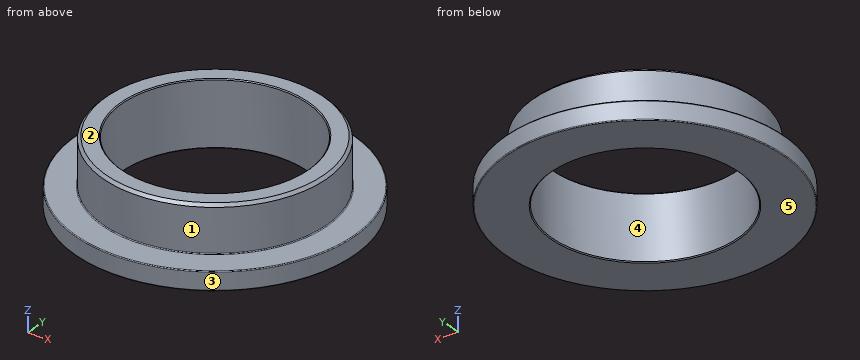
from build123d import *

# Parameters (mm, degrees)
CHAMFER1_SIZE = 0.15
CHAMFER2_SIZE = 0.05
FILLET1_R     = 0.045


with BuildPart() as part:
    # Sketch3 → Revolve1 (revolve)
    with BuildSketch(Plane(origin=(0, 0, 0), x_dir=(0, 0, -1), z_dir=(1, 0, 0))):
        Polygon((1.75, -7.5), (0.75, -7.5), (0.75, -6), (-1.75, -6), (-1.75, -5), (1.75, -5), align=None)
    revolve(axis=Axis((0, 0, 1.75), (0, 0, -1)))

    # Chamfer1
    chamfer1_edges = [part.edges().sort_by_distance(p)[0] for p in [
        (0, 6, 1.75),
    ]]
    chamfer(chamfer1_edges, length=CHAMFER1_SIZE)

    # Chamfer2
    chamfer2_edges = [part.edges().sort_by_distance(p)[0] for p in [
        (0, 5, -1.75),
        (0, 5, 1.75),
    ]]
    chamfer(chamfer2_edges, length=CHAMFER2_SIZE)

    # Fillet1
    fillet1_edges = [part.edges().sort_by_distance(p)[0] for p in [
        (0, 6, -0.75),
        (0, 7.5, -0.75),
        (0, 7.5, -1.75),
    ]]
    fillet(fillet1_edges, radius=FILLET1_R)


solid = part.part
The listing builds one solid part. Answer for the finished solid, in the listing's coordinates (mm). Face numbers are marked on the shaded views. A direction names the side the tool comes from. Give positions to 0.01 mm unless a question says otherwise; leave off trailing zeros. Order: outer loops, then holes, each group sorted by start corner. A loop starts at its lowest first (then second) coordinate and runs counter-clockwise, first axis right, second up. Notation, with made-up numbers: (-31, 45) - (-3, 45) arc R25 cw to (-3, 59) - close; hole circle Ø4 at (86.25, 65). An arc over 180 degrees is marked (long way). Use one line per item in the form item = value.
1) Find section D-D on z = -0.2. Determine the outline of the cut face in (x, y), and give its area (3 significant figures).
Verdict:
outline = circle Ø12 at (0, 0); hole circle Ø10 at (0, 0)
area = 34.6 mm^2
2) The mould has two halves that part along X. Classify the marked faces 3, 4 and 5: released by +X, released by -X, zero draft, split by the parting line, or undercut.
Verdict:
face_3 = split by the parting line
face_4 = undercut
face_5 = zero draft
3) Find section A-A on y = 0. Determine the outline of the cut face in (x, z) (3 decimals), and give its area (3 significant figures).
Verdict:
outline = (-7.5, -1.705) arc R0.045 ccw to (-7.455, -1.75) - (-5.05, -1.75) - (-5, -1.7) - (-5, 1.7) - (-5.05, 1.75) - (-5.85, 1.75) - (-6, 1.6) - (-6, -0.705) arc R0.045 cw to (-6.045, -0.75) - (-7.455, -0.75) arc R0.045 ccw to (-7.5, -0.795) - close; (5, -1.7) - (5.05, -1.75) - (7.455, -1.75) arc R0.045 ccw to (7.5, -1.705) - (7.5, -0.795) arc R0.045 ccw to (7.455, -0.75) - (6.045, -0.75) arc R0.045 cw to (6, -0.705) - (6, 1.6) - (5.85, 1.75) - (5.05, 1.75) - (5, 1.7) - close
area = 9.97 mm^2
4) Each of these flat-tipped pins is pushed along its axis until it touches: pin 1 (3 mm diameter, centred on x = -1, y = -4, fed in from +Z); pin 2 (2 mm diameter, centred on y = 3, z = -0.5, fed in from -X); pin 3 (2 mm diameter, centred on y = 1, z = 1, fed in from -X). Where does it stop, or does it pass through?
Verdict:
pin_1 = 1.75
pin_2 = -7.22
pin_3 = -6
5) For the marked faces 1 and 2, determine the directions among +Z, -Z, +X, -X, +Y, -Y from which every point of the face is accessible in a straight line to the end or side of a thin tool.
Verdict:
face_1 = +Z
face_2 = +Z, +X, -X, +Y, -Y
6) Find section C-C on z = -1. Determine the outline of the cut face in (x, y).
Verdict:
outline = circle Ø15 at (0, 0); hole circle Ø10 at (0, 0)
7) Consider probe 1 along X at (y, z) = (0, -0.25); probe 2 along X at (y, z) = (0, -0.8). Determine where each line is inside the solid, lowest interval first. Write a range as [from, to].
Verdict:
probe_1 = [-6, -5], [5, 6]
probe_2 = [-7.5, -5], [5, 7.5]
